The drawing under review shows one solid part. Ordinate dimensions are in mm from its lowest x, y, z. Round coordinates to 2 decimals unless told otherwise and drop trailing zeros. Write each loop counter-clockwise with the first axis right and the second up, starting at its lowest first coordinate (ties: lowest second). Pieces come first, ordered by that corner, then holes. Notation, with made-up numbers: M 4,-1 L 31,-1 A24 cw 31,30 Z; hole C 54,71.5 d2. An arc over 180 degrees is marked long. Write item = value, one per line. Start each with the question number.
Item 1: The part is to be moulded in two halves that separate along Z. For the marked faces 1, 2, 3 and 4, say which applies: +Z half, -Z half, draft (parallel to the pull), parting line (faces both ways), or undercut.
Item 2: Take a section at D-D, the plane x = 86. Give the boundary of the cut face in (y, z), plus the area to 3 significant figures.
Item 3: Take a section at B-B, the plane z = 30. Give the boundary of the cut face in (x, y), plus the area to 3 significant figures.
Item 4: Take a section at C-C, the plane y = 9.25. Give the number of separate pieces and of enclosed holes in the cut face, plus the area to 3 significant figures.
Item 5: To check wall thickness, follow line 1 along Z through (x, y) = (73.5, 4.5); line 2 along X through (y, z) = (7.75, 30); line 3 along X through (y, z) = (2, 32). State the ranges of each line that lie inside material, in increasing order.
Item 6: Take a section at A-A, the plane x = 6. Give the boundary of the cut face in (y, z).
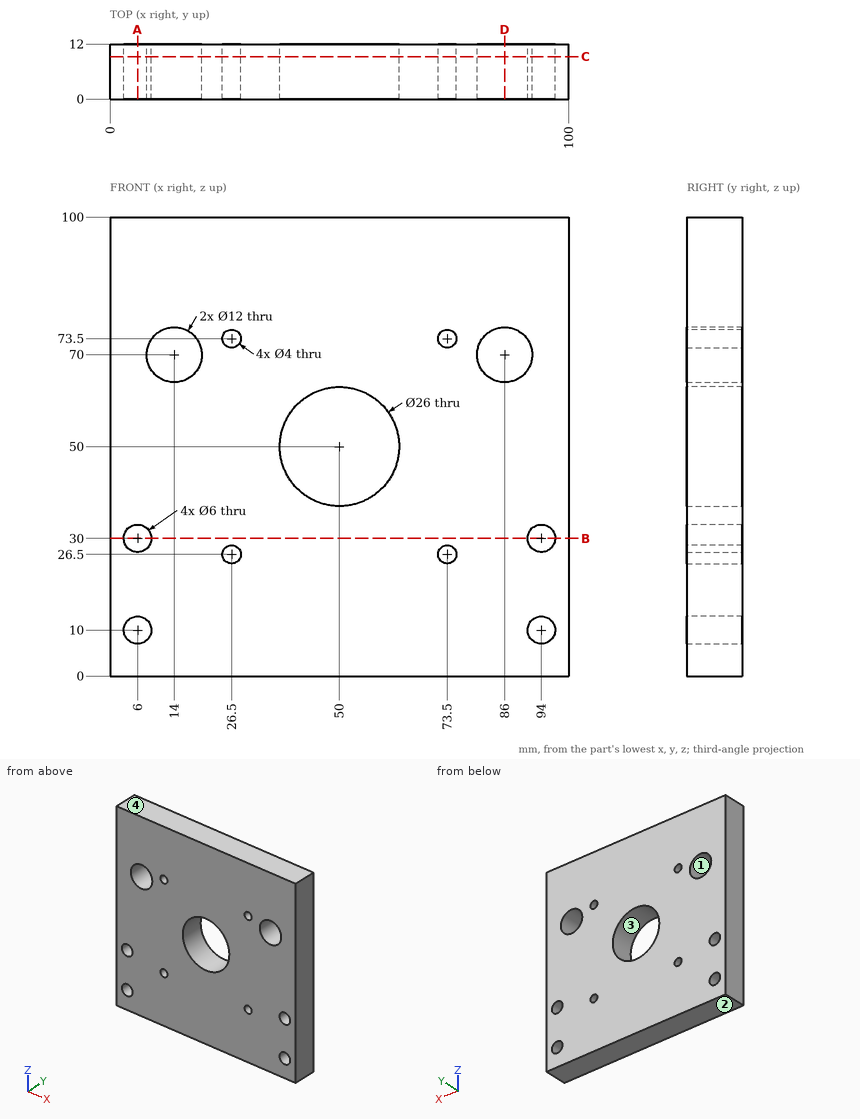
Response values:
q1.face_1 = undercut
q1.face_2 = -Z half
q1.face_3 = undercut
q1.face_4 = +Z half
q2.outline = M 0,0 L 12,0 L 12,64 L 0,64 Z; M 0,76 L 12,76 L 12,100 L 0,100 Z
q2.area = 1,060 mm2
q3.outline = M 0,0 L 3,0 L 3,12 L 0,12 Z; M 9,0 L 91,0 L 91,12 L 9,12 Z; M 97,0 L 100,0 L 100,12 L 97,12 Z
q3.area = 1,060 mm2
q4.separate_pieces = 1
q4.enclosed_holes = 11
q4.area = 9,080 mm2
q5.line_1 = 0 to 24.5, 28.5 to 71.5, 75.5 to 100
q5.line_2 = 0 to 3, 9 to 91, 97 to 100
q5.line_3 = 0 to 3.76, 8.24 to 91.76, 96.24 to 100
q6.outline = M 0,0 L 12,0 L 12,7 L 0,7 Z; M 0,13 L 12,13 L 12,27 L 0,27 Z; M 0,33 L 12,33 L 12,100 L 0,100 Z
